Drawing for the job (mm, zero at the part's lowest x, y, z). A direction names the side the tool comes from. Coordinates: 2 decimals unless noted, no trailing zeros. Write each loop counter-clockwise with the first axis right and the second up, starting at its lowest first coordinate (ties: lowest second). Pieces come first, ordered by that corner, then holes. Notation, with made-up numbers: (-6, 29) -> (36, 29) arc R14 ccw to (36, 40) -> close; hole circle Ø11 at (68, 66.25). An arc over 180 degrees is marked (long way). Answer as CSV lines item,"result".
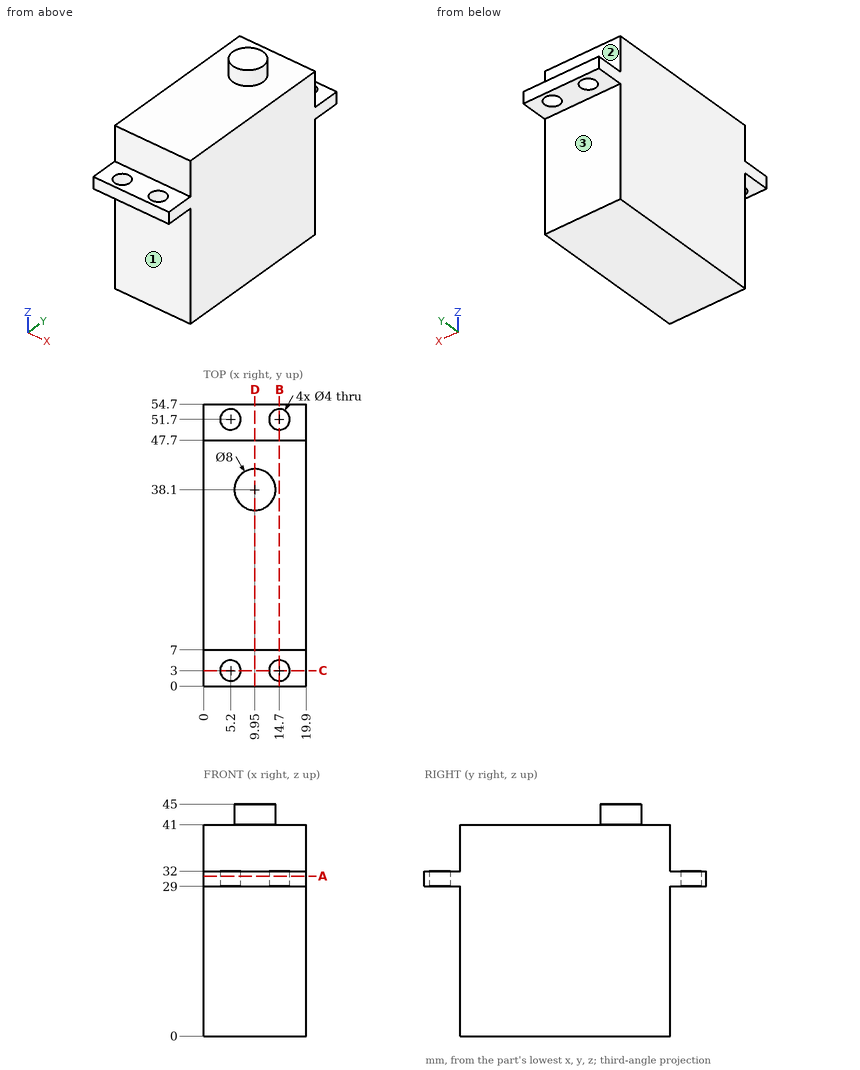
Item 1: Wall check: line 1 (Y direction, x = 14.7, z = 30.2); line 2 (X direction, y = 51, z = 30); line 3 (Z direction, x = 10.5, y = 6). Give the ranges that are in metal, low to high. Write a range as from..to.
Answer below:
line 1,"y = 0..1, 5..49.7, 53.7..54.7"
line 2,"x = 0..3.33, 7.07..12.83, 16.57..19.9"
line 3,"z = 29..32"
Item 2: Saw through at C-C on y = 3. Give the cut face in (x, z).
Answer below:
outline,"(0, 29) -> (3.2, 29) -> (3.2, 32) -> (0, 32) -> close; (7.2, 29) -> (12.7, 29) -> (12.7, 32) -> (7.2, 32) -> close; (16.7, 29) -> (19.9, 29) -> (19.9, 32) -> (16.7, 32) -> close"
Item 3: Flat gauge pins, fed straight in: pin 1 (5.5 mm diameter, centred on x = 5, y = 50.5, fed in from -Z); pin 2 (10 mm diameter, centred on x = 11, z = 38, fed in from -Y); pin 3 (10 mm diameter, centred on x = 7, z = 39.5, fed in from +Y). Where does each tip first touch, or does it go through?
Answer below:
pin 1,"stops at z = 29"
pin 2,"stops at y = 7"
pin 3,"stops at y = 47.7"
Item 4: 3-axis set-ups, long thin cutter, end or side, ignore diameter. For the marked faces 1, 2 and 3: which of +Z, -Z, +X, -X, +Y, -Y reach the whole face in a straight line?
Answer below:
face 1,"-Z, +X, -X, -Y"
face 2,"+Z, +X, -X, +Y"
face 3,"-Z, +X, -X, +Y"
Item 5: Saw through at B-B on x = 14.7. Give the cut face in (y, z).
Answer below:
outline,"(0, 29) -> (1, 29) -> (1, 32) -> (0, 32) -> close; (5, 29) -> (7, 29) -> (7, 0) -> (47.7, 0) -> (47.7, 29) -> (49.7, 29) -> (49.7, 32) -> (47.7, 32) -> (47.7, 41) -> (7, 41) -> (7, 32) -> (5, 32) -> close; (53.7, 29) -> (54.7, 29) -> (54.7, 32) -> (53.7, 32) -> close"
Item 6: Saw through at D-D on x = 9.95. Give the cut face in (y, z).
Answer below:
outline,"(0, 29) -> (7, 29) -> (7, 0) -> (47.7, 0) -> (47.7, 29) -> (54.7, 29) -> (54.7, 32) -> (47.7, 32) -> (47.7, 41) -> (42.1, 41) -> (42.1, 45) -> (34.1, 45) -> (34.1, 41) -> (7, 41) -> (7, 32) -> (0, 32) -> close"
Item 7: Saw through at A-A on z = 31. Give the cut face in (x, y), and give its area (3 significant figures).
Answer below:
outline,"(0, 0) -> (19.9, 0) -> (19.9, 54.7) -> (0, 54.7) -> close; hole circle Ø4 at (5.2, 3); hole circle Ø4 at (5.2, 51.7); hole circle Ø4 at (14.7, 3); hole circle Ø4 at (14.7, 51.7)"
area,"1,040 mm2"
